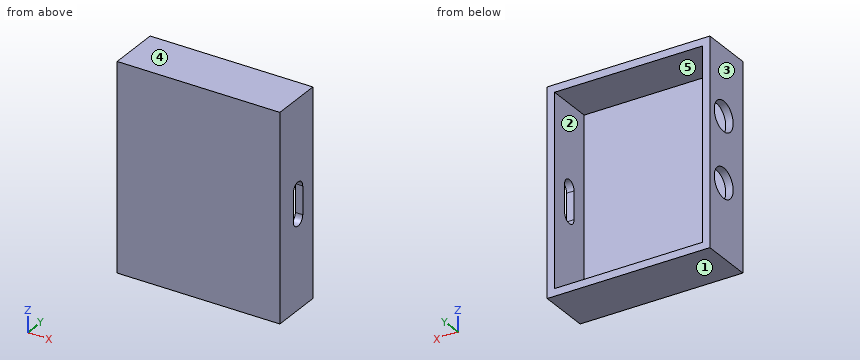
Autodesk Inventor part; units mm, degrees
ref_plane "YZ Plane" through (0, 0, 0) normal (1, 0, 0) x (0, 1, 0)
ref_plane "XZ Plane" through (0, 0, 0) normal (0, 1, 0) x (-1, 0, 0)
ref_plane "XY Plane" through (0, 0, 0) normal (0, 0, 1) x (1, 0, 0)
sketch "Sketch1" plane through (0, 0, 0) normal (0, 1, 0) x (-1, 0, 0)
  line L0 (-19.25, 24.25) -> (19.25, 24.25)
  line L1 (19.25, 24.25) -> (19.25, -24.25)
  line L2 (19.25, -24.25) -> (-19.25, -24.25)
  line L3 (-19.25, -24.25) -> (-19.25, 24.25)
  line L4 (-19.25, 24.25) -> (19.25, -24.25) construction
  line L5 (19.25, 24.25) -> (-19.25, -24.25) construction
  point P0 (0, 0)
  dimension "d0" = 38.5
  dimension "d1" = 48.5
extrude "Extrusion1" add sketch "Sketch1" along normal blind 12.25
sketch "Sketch2" plane through (0, 12.25, 0) normal (0, 1, 0) x (1, 0, 0)
  line L0 (-17.5, -22.5) -> (17.5, -22.5)
  line L1 (17.5, -22.5) -> (17.5, 22.5)
  line L2 (17.5, 22.5) -> (-17.5, 22.5)
  line L3 (-17.5, 22.5) -> (-17.5, -22.5)
  line L4 (-17.5, -22.5) -> (17.5, 22.5) construction
  line L5 (17.5, -22.5) -> (-17.5, 22.5) construction
  point P0 (0, 0)
  dimension "d4" = 35
  dimension "d5" = 45
extrude "Extrusion2" cut sketch "Sketch2" against normal blind 11
sketch "Sketch3" plane through (19.25, 0, 24.25) normal (1, 0, 0) x (0, 0, -1)
  line L0 (46.75, 1.25) -> (1.75, 1.25)
  line L1 (46.75, 12.25) -> (46.75, 1.25)
  line L2 (1.75, 12.25) -> (1.75, 1.25)
  line L3 (1.75, 8.5) -> (19.15, 8.5)
  line L4 (46.75, 8.5) -> (29.25, 8.5)
  line L5 (19.15, 1.25) -> (19.15, 5)
  line L6 (19.15, 5) -> (29.25, 5)
  line L7 (29.25, 5) -> (29.25, 8.5)
  line L8 (29.25, 8.5) -> (19.15, 8.5)
  line L9 (19.15, 8.5) -> (19.15, 5)
  circle A0 centre (20.9, 6.75) radius 1.75
  circle A1 centre (27.5, 6.75) radius 1.75
  point P0 (24.25, 0)
  point P1 (20.9, 5)
  point P2 (27.5, 5)
  point P3 (27.5, 8.5)
  point P4 (20.9, 8.5)
  dimension "d8" = 17.4
  dimension "d9" = 17.5
  dimension "d10" = 3.75
  dimension "d11" = 3.75
  dimension "d12" = 3.75
  dimension "d22" = 0
extrude "Extrusion3" cut sketch "Sketch3" against normal blind 11 contours A0 L8 A1 L6 | A0 | A1
sketch "Sketch4" plane through (-19.25, 0, -24.25) normal (-1, 0, 0) x (0, 0, 1)
  line L0 (46.75, 1.25) -> (1.75, 1.25)
  line L1 (1.75, 12.25) -> (1.75, 1.25)
  line L2 (46.75, 12.25) -> (46.75, 1.25)
  line L3 (24.25, 1.25) -> (24.25, 6.36)
  line L4 (1.75, 7.11) -> (17.25, 7.11)
  line L5 (46.75, 7.11) -> (32.55, 7.11)
  circle A0 centre (17.25, 7.11) radius 3.504
  circle A1 centre (32.55, 7.11) radius 3.504
  point P0 (24.25, 0)
  dimension "d23" = 5.11
  dimension "d24" = 15.5
  dimension "d25" = 14.2
extrude "Extrusion4" cut sketch "Sketch4" against normal blind 11
The listing builds one solid part. Answer for the finished solid, in the listing's coordinates (mm). Face numbers are marked on the shaded views. A direction names the side the tool comes from. Give positions to 0.01 mm unless a question says otherwise; leave off trailing zeros. Order: outer loops, then holes, each group sorted by start corner. A loop starts at its lowest first (then second) coordinate and runs counter-clockwise, first axis right, second up. Notation, with made-up numbers: (-15.5, -10) - (-0.5, -10) arc R8 ccw to (-0.5, -5) - close; hole circle Ø7 at (-35.75, -23.5). An arc over 180 degrees is marked (long way). One line per item, written item: value. Start each with the question number.
1) Find the intervals of material crossed by L1, parallel to X at y = 3.25, z = 4.5; L2, parallel to Z at x = 7, y = 10.75; L3, parallel to Y at x = -18.35, z = -7, in increasing order.
2) A cutting plane is placed at B-B on z = -14.5. Give the vertices of the cut face in (x, y).
3) A cutting plane is placed at C-C on y = 11.25. Give the vertices of the cut face in (x, z), then the cut area to 3 significant figures.
4) A cutting plane is placed at D-D on x = -0.5. Give the vertices of the cut face in (y, z).
5) The mould has two halves that part along Z. Classify the marked faces 3, 4 and 5: released by +Z, released by -Z, zero draft, split by the parting line, or undercut.
6) A tool of negligible diameter and unlimited length cuts with its end or side. For the marked faces 1 and 2, from which of +Z, -Z, +X, -X, +Y, -Y can it reach the whole face along a straight path? Write none if from no direction.
7) Given pin 1 Ø10.5 at (x, z) = (-1.5, 8.5) entering from +Y, flat-ended and moving along its own axis, determine where the tip first touches the part or whether it passes through.
8) A cutting plane is placed at A-A on z = 8.3. Give the vertices of the cut face in (x, y), then the cut area to 3 significant figures.
Answer sheet:
1. L1: x = -19.25 to -17.5, 17.5 to 19.25
1. L2: z = -24.25 to -22.5, 22.5 to 24.25
1. L3: y = 0 to 3.61, 10.61 to 12.25
2. outline: (-19.25, 0) - (19.25, 0) - (19.25, 12.25) - (17.5, 12.25) - (17.5, 1.25) - (-17.5, 1.25) - (-17.5, 12.25) - (-19.25, 12.25) - close
3. outline: (-19.25, -24.25) - (19.25, -24.25) - (19.25, 24.25) - (-19.25, 24.25) - close; hole (-17.5, -22.5) - (17.5, -22.5) - (17.5, 22.5) - (-17.5, 22.5) - close
3. area: 292 mm2
4. outline: (0, -24.25) - (12.25, -24.25) - (12.25, -22.5) - (1.25, -22.5) - (1.25, 22.5) - (12.25, 22.5) - (12.25, 24.25) - (0, 24.25) - close
5. face 3: zero draft
5. face 4: released by +Z
5. face 5: undercut
6. face 1: -Z, +X, -X, +Y, -Y
6. face 2: +Y
7. pin 1: stops at y = 1.25
8. outline: (-19.25, 0) - (19.25, 0) - (19.25, 12.25) - (17.5, 12.25) - (17.5, 1.25) - (-17.5, 1.25) - (-17.5, 3.61) - (-19.25, 3.61) - close; (-19.25, 10.61) - (-17.5, 10.61) - (-17.5, 12.25) - (-19.25, 12.25) - close
8. area: 74.4 mm2
